```python
from build123d import *

# Parameters (mm, degrees)
F1_DEPTH = 82.55
F3_R     = 4.3688
F4_DEPTH = 25.4
F5_DEPTH = 25.4


with BuildPart() as f1:
    # F0 (on Front) → F1 (new body)
    with BuildSketch(Plane.XZ):
        Polygon((-38.1, 0), (0, 0), (0, 153.3652), (-18.0848, 153.3652), (-38.1, 133.35), align=None)
    extrude(amount=F1_DEPTH)

    # F3 (on face) → F4 (cut)
    with BuildSketch(Plane(origin=(0, 0, 0), x_dir=(1, 0, 0), z_dir=(0, 0, -1))):
        with Locations((-19.05, 9.525)):
            Circle(F3_R)
        with Locations((-19.05, 73.025)):
            Circle(F3_R)
    extrude(amount=-F4_DEPTH, mode=Mode.SUBTRACT)

    # F2 (on face) → F5 (cut)
    with BuildSketch(Plane(origin=(-85.725, 0, 85.725), x_dir=(0, -1, 0), z_dir=(-0.707107, 0, 0.707107))):
        with BuildLine():
            ThreePointArc((68.6562, 81.504805), (73.025, 77.136005), (77.3938, 81.504805))
            Line((77.3938, 81.504805), (73.025, 81.504805))
            Line((73.025, 81.504805), (68.6562, 81.504805))
        make_face()
        with BuildLine():
            Line((73.025, 81.504805), (77.3938, 81.504805))
            ThreePointArc((77.3938, 81.504805), (73.025, 85.873605), (68.6562, 81.504805))
            Line((68.6562, 81.504805), (73.025, 81.504805))
        make_face()
        with BuildLine():
            ThreePointArc((5.1562, 81.504805), (9.525, 77.136005), (13.8938, 81.504805))
            Line((13.8938, 81.504805), (9.525, 81.504805))
            Line((9.525, 81.504805), (5.1562, 81.504805))
        make_face()
        with BuildLine():
            Line((9.525, 81.504805), (13.8938, 81.504805))
            ThreePointArc((13.8938, 81.504805), (9.525, 85.873605), (5.1562, 81.504805))
            Line((5.1562, 81.504805), (9.525, 81.504805))
        make_face()
    extrude(amount=-F5_DEPTH, mode=Mode.SUBTRACT)


solid = f1.part
```
Build history of the part. All positions in model axes, mm. A direction names the side the tool comes from. Give positions to 0.01 mm unless a question says otherwise; leave off trailing zeros. Loops run counter-clockwise (first coordinate to the right, second up) from the corner with the lowest first, then second, coordinate; pieces in that order, holes last.
1) Drop flat-ended pins along their axis: P1, Ø4, axis at y = -19.5, z = 63, coming from the +X side; P2, Ø8, axis at x = -19.05, y = -73.025, coming from the -Z side. Give the stop position or say it passes through.
Values follow:
P1: stops at x = 0
P2: stops at z = 25.4
2) 3-axis set-ups, long thin cutter, end or side, ignore diameter. For faces 5 (the face through (-10.09, -72.96, 125.44)), 6 (the face through (0, -41, 76)), 7 (the face through (-19, -10, 25.4)): which of +Z, -Z, +X, -X, +Y, -Y reach the whole face in a straight line?
Values follow:
face 5: none
face 6: +Z, -Z, +X, +Y, -Y
face 7: -Z
3) Probe line 1 along Y through (x, z) = (-19, 20); line 2 along Y through (x, z) = (-26, 144); line 3 along Z through (x, y) = (-25, -49). List the from-to ranges inside material, lowest first.
Values follow:
line 1: y = -82.55 to -77.39, -68.66 to -13.89, -5.16 to 0
line 2: y = -82.55 to -76.94, -69.11 to -13.44, -5.61 to 0
line 3: z = 0 to 146.45
4) Two-plate mould, pull along X, no slides. Class faces 1 (the face through (-19, -41, 0)), 2 (the face through (-16.2, -9, 137.6)), 3 (the face through (-27.95, -40.7, 143.5)), 4 (the face through (-14.883, -10.837, 12.522)): released by +X, released by -X, zero draft, split by the parting line, or undercut.
Values follow:
face 1: zero draft
face 2: undercut
face 3: released by -X
face 4: undercut
5) Band-saw the part on B-B on z = 10. List the corners of the cut face in (x, y) (3 decimals).
Values follow:
outline: (-38.1, -82.55) - (0, -82.55) - (0, 0) - (-38.1, 0) - close; hole circle Ø8.738 at (-19.05, -73.025); hole circle Ø8.738 at (-19.05, -9.525)
6) Band-saw the part on A-A on y = -59. List the corners of the cut face in (x, z).
Values follow:
outline: (-38.1, 0) - (0, 0) - (0, 153.37) - (-18.08, 153.37) - (-38.1, 133.35) - close
